```python
from build123d import *

# Parameters (mm, degrees)
F0_R     = 15
F1_DEPTH = 30
F2_R     = 10
F3_DEPTH = 30.001
F4_R     = 5
F5_DEPTH = 25


with BuildPart() as f1:
    # F0 (on Right) → F1 (new body)
    with BuildSketch(Plane.YZ):
        with BuildLine():
            Line((52.862198, 14.724396), (0, 25))
            ThreePointArc((0, 25), (-25, 0), (0, -25))
            Line((0, -25), (50, -15))
            ThreePointArc((50, -15), (64.93094, -1.437718), (52.862198, 14.724396))
        make_face()
        Circle(F0_R, mode=Mode.SUBTRACT)
    extrude(amount=F1_DEPTH)

    # F2 (on face) → F3 (cut, through all)
    with BuildSketch(Plane.YZ.offset(30)):
        with Locations((50, 0)):
            Circle(F2_R)
    extrude(amount=-F3_DEPTH, mode=Mode.SUBTRACT)

    # F4 (on face) → F5 (cut)
    with BuildSketch(Plane.YZ.offset(30)):
        with Locations((23.703395, 14.439134)):
            Circle(F4_R)
    extrude(amount=-F5_DEPTH, mode=Mode.SUBTRACT)


solid = f1.part
```
Geometry check sheet. Reference: the model listing, model coordinates, mm. A direction names the side the tool comes from. Give positions to 0.01 mm unless a question says otherwise; leave off trailing zeros. Loops run counter-clockwise (first coordinate to the right, second up) from the corner with the lowest first, then second, coordinate; pieces in that order, holes last. Notation, with made-up numbers: M -19.5,-16.5 L 1.5,-16.5 A24 ccw 1.5,-6.5 Z; hole C 14.25,73.25 d6. An arc over 180 degrees is marked long. Write item = value, one per line. Start each with the question number.
1. Section check D-D, the plane x = 13.25. Enter the section's corners in (y, z), plus the area to 3 significant figures.
2. Thickness scan on probe 1 along Y at (x, z) = (11.5, 8.5); probe 2 along Y at (x, z) = (27, 1); probe 3 along Z at (x, y) = (12.25, 0). Record the ranges inside material, lowest first.
3. Section check C-C, the plane y = 12. Enter the section's corners in (x, z), plus the area to 3 significant figures.
4. Go/stop test with flat-tipped pins: P1, Ø6, axis at y = 23.7, z = 14.44, coming from the +X side; P2, Ø6, axis at x = 24.5, y = 27.5, coming from the +Z side; P3, Ø12, axis at x = 23.5, y = 26, coming from the -Z side. Record where each tip stops, or that it passes through.
5. Draft check along Z on faces 1 (the face through (14.79, -24.994, 0.55)), 2 (the face through (14.79, -14.985, 0.66)), 3 (the face through (17.675, 22.619, 9.558)), 4 (the face through (0, 19, 0)). Enter one of: +Z half, -Z half, draft (parallel to the pull), parting line (faces both ways), or undercut.
6. Section check B-B, the plane x = 2.5. Enter the section's corners in (y, z).
7. Tool access check on faces 5 (the face through (5, 24, 15)), 6 (the face through (14.79, 26.8, 19.79)). Record the directions out of +Z, -Z, +X, -X, +Y, -Y that give a thin tool (end or side, any length) a straight path to the whole face; none if there is none.
8. Section check A-A, the plane z = -8.5. Enter the section's corners in (x, y), plus the area to 3 significant figures.
Values follow:
q1.outline = M 0,-25 L 50,-15 A15 ccw 52.86,14.72 L 0,25 A25 ccw Z; hole C 0,0 d30; hole C 23.7,14.44 d10; hole C 50,0 d20
q1.area = 2,240 mm^2
q2.probe_1 = -23.51 to -12.36, 12.36 to 44.73, 55.27 to 62.36
q2.probe_2 = -24.98 to -14.97, 14.97 to 40.05, 59.95 to 64.97
q2.probe_3 = -25 to -15, 15 to 25
q3.outline = M 0,-22.6 L 30,-22.6 L 30,-9 L 0,-9 Z; M 0,9 L 30,9 L 30,22.67 L 0,22.67 Z
q3.area = 818 mm^2
q4.P1 = 5
q4.P2 = 20.24
q4.P3 = -21
q5.face_1 = parting line
q5.face_2 = undercut
q5.face_3 = undercut
q5.face_4 = draft
q6.outline = M 0,-25 L 50,-15 A15 ccw 52.86,14.72 L 0,25 A25 ccw Z; hole C 0,0 d30; hole C 50,0 d20
q7.face_5 = +X
q7.face_6 = +Z, +X, -X, +Y
q8.outline = M 0,-23.51 L 30,-23.51 L 30,-12.36 L 0,-12.36 Z; M 0,12.36 L 30,12.36 L 30,44.73 L 0,44.73 Z; M 0,55.27 L 30,55.27 L 30,62.36 L 0,62.36 Z
q8.area = 1,520 mm^2
